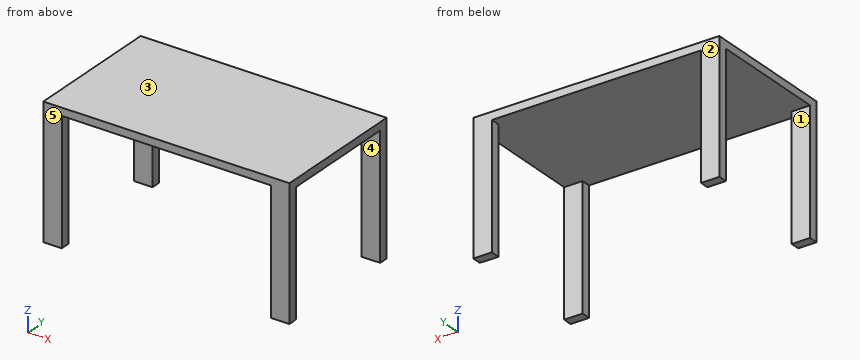
```python
from build123d import *

# Parameters (mm, degrees)
F0_W     = 1600
F0_H     = 900
F1_DEPTH = 50
F2_W     = 120
F2_H     = 60
F3_DEPTH = 800


# Not quite as in the source:
# - a pattern or mirror of a feature is missing from the dataset's text; its kind, count and spacing are read off the source's solid


with BuildPart() as f1:
    # F0 (on Top) → F1 (new body)
    with BuildSketch(Plane.XY):
        Rectangle(F0_W, F0_H)
    extrude(amount=F1_DEPTH)

    # F2 (on face) → F3 (join)
    with BuildSketch(Plane(origin=(0, 0, 0), x_dir=(1, 0, 0), z_dir=(0, 0, -1))):
        with Locations((-740, 420)):
            Rectangle(F2_W, F2_H)
        with Locations((-740, -420)):
            Rectangle(F2_W, F2_H)
    f3 = extrude(amount=F3_DEPTH)

    # F3_copies: F3 across plane
    add(f3.mirror(Plane(origin=(0, 0, 0), x_dir=(0, 0, 1), z_dir=(1, 0, 0))))


solid = f1.part
```
Could you check a few things on this model? Use its own coordinates, in mm. Face numbers are marked on the shaded views. A direction names the side the tool comes from. Round coordinates to 2 decimals unless told otherwise and drop trailing zeros. Loops run counter-clockwise (first coordinate to the right, second up) from the corner with the lowest first, then second, coordinate; pieces in that order, holes last. Notation, with made-up numbers: (41, 40) - (76, 40) arc R29 ccw to (76, 76) - close; hole circle Ø1 at (52.25, 18). An arc over 180 degrees is marked (long way). Answer as CSV lines item,"result".
1. For pin 1 Ø8 at (x, y) = (-555, 281.5) entering from -Z, with a flat end and sliding along its axis, tell me the tip position at first contact or that it passes through.
Filled in:
pin 1,"stops at z = 0"
2. Please list where these lines run through material, in increasing order: line 1 along Y through (x, z) = (-689, -441.5); line 2 along X through (y, z) = (-406.5, -23.5); line 3 along Z through (x, y) = (210, 402). Write a range as [from, to].
Filled in:
line 1,"y = [-450, -390], [390, 450]"
line 2,"x = [-800, -680], [680, 800]"
line 3,"z = [0, 50]"
3. I want a section at C-C on y = -33. List the corners of the cut face in (x, z) for me, then the cut area to 3 significant figures.
Filled in:
outline,"(-800, 0) - (800, 0) - (800, 50) - (-800, 50) - close"
area,"80,000 mm^2"
4. On a 3-axis mill with a long thin cutter (end or side, diameter ignored), from which of +Z, -Z, +X, -X, +Y, -Y can I reach the whole of each face in a straight line? I mean the marked faces 1 and 2. Say none if no direction works.
Filled in:
face 1,"-Z, +X, -X"
face 2,"+Z, -Z, +X, -X, +Y"
5. I want a section at A-A on z = -362. List the corners of the cut face in (x, y) for me, then the cut area to 3 significant figures.
Filled in:
outline,"(-800, -450) - (-680, -450) - (-680, -390) - (-800, -390) - close; (-800, 390) - (-680, 390) - (-680, 450) - (-800, 450) - close; (680, -450) - (800, -450) - (800, -390) - (680, -390) - close; (680, 390) - (800, 390) - (800, 450) - (680, 450) - close"
area,"28,800 mm^2"
6. I want a section at B-B on x = 63. List the corners of the cut face in (y, z) for me.
Filled in:
outline,"(-450, 0) - (450, 0) - (450, 50) - (-450, 50) - close"
7. We'd pull the mould along Y, two halves only. Please class the marked faces 3, 4 and 5: +Y half, -Y half, draft (parallel to the pull), parting line (faces both ways), or undercut.
Filled in:
face 3,"draft"
face 4,"undercut"
face 5,"-Y half"
